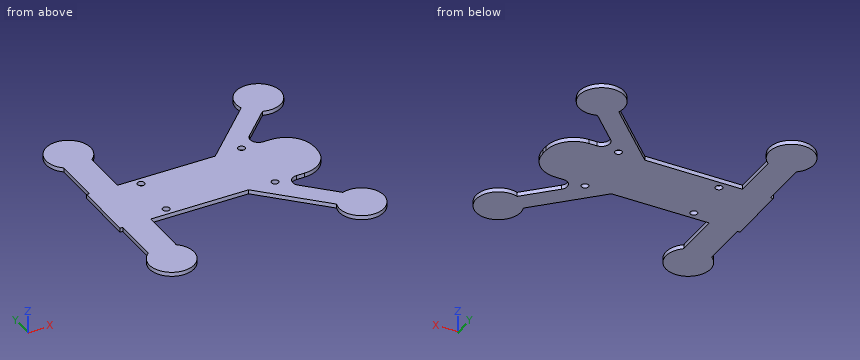
```python
from build123d import *

# Parameters (mm, degrees)
F1_DEPTH = 1.5
F2_R     = 1.25
F3_DEPTH = 25


with BuildPart() as f1:
    # F0 (on Top) → F1 (new body)
    with BuildSketch(Plane.XY):
        with BuildLine():
            Line((-7, 11), (-7, 27.755002))
            ThreePointArc((-7, 27.755002), (-12, 42), (-17, 27.755002))
            Line((-17, 27.755002), (-17, 11))
            Line((-17, 11), (-18, 11))
            Line((-18, 11), (-18, -11))
            Line((-18, -11), (-17, -11))
            Line((-17, -11), (-17, -27.755002))
            ThreePointArc((-17, -27.755002), (-12, -42), (-7, -27.755002))
            Line((-7, -27.755002), (-7, -11))
            Line((-7, -11), (28.050253, -11))
            Line((28.050253, -11), (48.438379, -31.388126))
            ThreePointArc((48.438379, -31.388126), (61.656854, -39.656854), (53.388126, -26.438379))
            Line((53.388126, -26.438379), (43.071068, -16.12132))
            ThreePointArc((43.071068, -16.12132), (42.42075, -12.85195), (45.192388, -11))
            Line((45.192388, -11), (48, -11))
            ThreePointArc((48, -11), (55.071068, -8.071068), (58, -1))
            Line((58, -1), (58, 1))
            ThreePointArc((58, 1), (55.071068, 8.071068), (48, 11))
            Line((48, 11), (45.192388, 11))
            ThreePointArc((45.192388, 11), (42.42075, 12.85195), (43.071068, 16.12132))
            Line((43.071068, 16.12132), (53.388126, 26.438379))
            ThreePointArc((53.388126, 26.438379), (61.656854, 39.656854), (48.438379, 31.388126))
            Line((48.438379, 31.388126), (28.050253, 11))
            Line((28.050253, 11), (-7, 11))
        make_face()
    extrude(amount=F1_DEPTH)

    # F2 (on Top) → F3 (cut)
    with BuildSketch(Plane.XY):
        with Locations((0, -8.25)):
            Circle(F2_R)
        with Locations((0, 8.25)):
            Circle(F2_R)
        with Locations((37.5, -11)):
            Circle(F2_R)
        with Locations((37.5, 11)):
            Circle(F2_R)
    extrude(amount=F3_DEPTH, mode=Mode.SUBTRACT)


solid = f1.part
```
Part model, mm, in its own coordinate system. Round coordinates to 2 decimals unless told otherwise and drop trailing zeros. Loops run counter-clockwise (first coordinate to the right, second up) from the corner with the lowest first, then second, coordinate; pieces in that order, holes last. Notation, with made-up numbers: (42, 84) -> (80, 84) arc R8 cw to (80, 95) -> close; hole circle Ø4 at (33, -14.75). An arc over 180 degrees is marked (long way). Use CSV: the item, a comma, the result in double quotes. Start each with the question number.
1) Cut at D-D, the plane y = 34. Write the cut outline in (x, z).
2) Cut at A-A, the plane x = 0. Write the cut outline in (y, z), plus the area to 3 significant figures.
3) Drop flat-ended pins along their axis: P1, Ø2, axis at x = 37.5, y = -11, coming from the -Z side; P2, Ø0.8, axis at x = 46, z = 0.5, coming from the +Y side; P3, Ø0.8, axis at y = -18.5, z = 0.5, coming from the +X side; P4, Ø10, axis at x = 12, y = 14.5, coming from the +Z side. Give the stop position or say it passes through.
4) Wall check: L1, parallel to Y at x = 0, z = 0.75; L2, parallel to Y at x = 37.5, z = 0.55; L3, parallel to Y at x = 11, z = 0.95. Give the ranges that are in metal, low to high. Write a range as [from, to].
5) Cut at B-B, the plane y = 8.25. Write the cut outline in (x, z).
6) Cut at C-C, the plane z = 1.1. Write the cut outline in (x, y) (3 decimals), plus the area to 3 significant figures.
Determined:
1,outline,"(-20, 0) -> (-4, 0) -> (-4, 1.5) -> (-20, 1.5) -> close; (48, 0) -> (64, 0) -> (64, 1.5) -> (48, 1.5) -> close"
2,outline,"(-11, 0) -> (-9.5, 0) -> (-9.5, 1.5) -> (-11, 1.5) -> close; (-7, 0) -> (7, 0) -> (7, 1.5) -> (-7, 1.5) -> close; (9.5, 0) -> (11, 0) -> (11, 1.5) -> (9.5, 1.5) -> close"
2,area,"25.5 mm2"
3,P1,"passes through"
3,P2,"stops at y = 29.35"
3,P3,"stops at x = 45.85"
3,P4,"stops at z = 1.5"
4,L1,"y = [-11, -9.5], [-7, 7], [9.5, 11]"
4,L2,"y = [-20.45, -12.25], [-9.75, 9.75], [12.25, 20.45]"
4,L3,"y = [-11, 11]"
5,outline,"(-18, 0) -> (-1.25, 0) -> (-1.25, 1.5) -> (-18, 1.5) -> close; (1.25, 0) -> (54.89, 0) -> (54.89, 1.5) -> (1.25, 1.5) -> close"
6,outline,"(-18, -11) -> (-17, -11) -> (-17, -27.755) arc R8 ccw (long way) to (-7, -27.755) -> (-7, -11) -> (28.05, -11) -> (48.438, -31.388) arc R8 ccw (long way) to (53.388, -26.438) -> (43.071, -16.121) arc R3 cw to (45.192, -11) -> (48, -11) arc R10 ccw to (58, -1) -> (58, 1) arc R10 ccw to (48, 11) -> (45.192, 11) arc R3 cw to (43.071, 16.121) -> (53.388, 26.438) arc R8 ccw (long way) to (48.438, 31.388) -> (28.05, 11) -> (-7, 11) -> (-7, 27.755) arc R8 ccw (long way) to (-17, 27.755) -> (-17, 11) -> (-18, 11) -> close; hole circle Ø2.5 at (0, -8.25); hole circle Ø2.5 at (0, 8.25); hole circle Ø2.5 at (37.5, -11); hole circle Ø2.5 at (37.5, 11)"
6,area,"3,090 mm2"
